Here's how the part is built. I have some questions about the finished solid (model axes, mm). A direction names the side the tool comes from. Give positions to 0.01 mm unless a question says otherwise; leave off trailing zeros. Loops run counter-clockwise (first coordinate to the right, second up) from the corner with the lowest first, then second, coordinate; pieces in that order, holes last. Notation, with made-up numbers: (33.25, 10) - (77.25, 10) arc R19 ccw to (77.25, 18) - close; hole circle Ø9 at (80.5, -34.5). An arc over 180 degrees is marked (long way). Return JSON: item names as keys, results as strings. Group by question number.
(1) On a 3-axis mill with a long thin cutter (end or side, diameter ignored), from which of +Z, -Z, +X, -X, +Y, -Y can I reach the whole of each face in a straight line? I mean faces 1 (the flat face through (5.3, -0.5, 5.4)), 2 (the flat face through (12.5, -0.5, 5.4)). Say none if no direction works.
(2) If we section it at B-B (x = 7.75): Please give me the cut outline in (y, z), then the cut area to 3 significant figures.
(3) I need wall thicknesses on probe 1 along Z at (x, y) = (9.25, -0.45); probe 2 along Z at (x, y) = (9, -0.4); probe 3 along Z at (x, y) = (4.5, -0.85). Which ranges of each line are inside material? Lowest first, please. Write a range as [from, to].
(4) If we section it at A-A (z = 9.5): State how many separate pieces and enclosed holes the cut face has, then the cut area to 3 significant figures.
(5) If we section it at D-D (x = 3): Please give me the cut outline in (y, z).
(6) For P1, Ø0.5, axis at x = 9.5, y = -0.5, coming from the -Z side, with a flat end and sliding along its axis, tell me the tip position at first contact or that it passes through.
(7) If we mould it in two halves opening along Z, with no side actions, what happens to faces 3 (the flat face through (5.85, -0.5, 5.4)), 4 (the flat face through (6.93, -0.49, 12.48)), 5 (the flat face through (6.2, -0.5, 0))? For each: released by +Z, released by -Z, zero draft, split by the parting line, or undercut.
```python
from build123d import *

# Parameters (mm, degrees)
F0_W     = 1.05
F0_H     = 9
F0_W_2   = 1
F1_DEPTH = 1


with BuildPart() as f1:
    # F0 (on Front) → F1 (new body)
    with BuildSketch(Plane.XZ):
        Polygon((0, 14), (0, 0), (12.5, 0), (12.5, 11), (1.2, 14), (0.897396, 15), (0.302604, 15), align=None)
        with Locations((1.725, 5.5)):
            Rectangle(F0_W, F0_H, mode=Mode.SUBTRACT)
        with Locations((3.25, 5.5)):
            Rectangle(F0_W_2, F0_H, mode=Mode.SUBTRACT)
        with Locations((4.8, 5.5)):
            Rectangle(F0_W_2, F0_H, mode=Mode.SUBTRACT)
        with Locations((6.35, 5.5)):
            Rectangle(F0_W_2, F0_H, mode=Mode.SUBTRACT)
        with Locations((7.9, 5.5)):
            Rectangle(F0_W_2, F0_H, mode=Mode.SUBTRACT)
        with Locations((9.45, 5.5)):
            Rectangle(F0_W_2, F0_H, mode=Mode.SUBTRACT)
        with Locations((11, 5.5)):
            Rectangle(F0_W_2, F0_H, mode=Mode.SUBTRACT)
        Polygon((5.046939, 12.461368), (1.2, 11), (3.413901, 12.894918), align=None, mode=Mode.SUBTRACT)
        Polygon((1.2, 11.65814), (1.2, 13.482679), (2.827012, 13.050729), align=None, mode=Mode.SUBTRACT)
        Polygon((5.875713, 12.24134), (10.551425, 11), (2.607982, 11), align=None, mode=Mode.SUBTRACT)
    extrude(amount=F1_DEPTH)


solid = f1.part
```
Values:
{
 "1": {"face 1": "+Y, -Y", "face 2": "+Z, -Z, +X, +Y, -Y"},
 "2": {"outline": "(-1, 0) - (0, 0) - (0, 1) - (-1, 1) - close; (-1, 10) - (0, 10) - (0, 11) - (-1, 11) - close; (-1, 11.74) - (0, 11.74) - (0, 12.26) - (-1, 12.26) - close", "area": "2.52 mm2"},
 "3": {"probe 1": "[0, 1], [10, 11], [11.35, 11.86]", "probe 2": "[0, 1], [10, 11], [11.41, 11.93]", "probe 3": "[0, 1], [10, 11], [11.72, 12.25], [12.61, 13.12]"},
 "4": {"separate pieces": "8", "enclosed holes": "0", "area": "5.45 mm2"},
 "5": {"outline": "(-1, 0) - (0, 0) - (0, 1) - (-1, 1) - close; (-1, 10) - (0, 10) - (0, 11) - (-1, 11) - close; (-1, 11.15) - (0, 11.15) - (0, 11.68) - (-1, 11.68) - close; (-1, 12.54) - (0, 12.54) - (0, 13.52) - (-1, 13.52) - close"},
 "6": {"P1": "z = 0"},
 "7": {"face 3": "undercut", "face 4": "released by +Z", "face 5": "released by -Z"}
}
